Autodesk Inventor part; units mm, degrees
ref_plane "YZ Plane" through (0, 0, 0) normal (1, 0, 0) x (0, 1, 0)
ref_plane "XZ Plane" through (0, 0, 0) normal (0, 1, 0) x (-1, 0, 0)
ref_plane "XY Plane" through (0, 0, 0) normal (0, 0, 1) x (1, 0, 0)
sketch "Skizze1" plane through (0, 0, 0) normal (0, 1, 0) x (-1, 0, 0)
  line L0 (0, 0) -> (32, 0)
  line L1 (32, 0) -> (32, 5)
  line L2 (32, 5) -> (0, 5)
  line L3 (0, 5) -> (0, 0)
  dimension "d0" = 32
  dimension "d1" = 5
extrude "Extrusion1" add sketch "Skizze1" along normal blind 2
ref_plane "Arbeitsebene1" through (-32, 0, 2.5) normal (0, 0, 1) x (1, 0, 0)
ref_plane "Arbeitsebene2" through (-16, 0, 5) normal (1, 0, 0) x (0, 0, -1)
sketch "Skizze2" plane through (0, 2, 0) normal (0, 1, 0) x (1, 0, 0)
  line L0 (6.4, -2.5) -> (-38.4, -2.5)
  line L1 (-16, 1) -> (-16, -6)
  point P0 (0, 0)
  point P1 (-28.5, -2.5)
  point P2 (-16, -2.5)
  point P3 (-3.5, -2.5)
  dimension "d4" = 25
  dimension "d5" = 12.5
hole "Bohrung1" at (-28.5, 2, 2.5) at (-16, 2, 2.5) at (-3.5, 2, 2.5) direction (0, -1, 0) diameter 3.2 end through all
sketch "Skizze3" plane through (0, 2, 0) normal (0, 1, 0) x (1, 0, 0)
  line L0 (-18, -4.75) -> (-25, -4.75)
  line L1 (-25, -4.75) -> (-25, -4.25)
  line L2 (-25, -4.25) -> (-18, -4.25)
  line L3 (-18, -4.25) -> (-18, -4.75)
  line L4 (-18, -3.75) -> (-25, -3.75)
  line L5 (-25, -3.75) -> (-25, -3.25)
  line L6 (-25, -3.25) -> (-18, -3.25)
  line L7 (-18, -3.25) -> (-18, -3.75)
  line L8 (-18, -2.75) -> (-25, -2.75)
  line L9 (-25, -2.75) -> (-25, -2.25)
  line L10 (-25, -2.25) -> (-18, -2.25)
  line L11 (-18, -2.25) -> (-18, -2.75)
  line L12 (-18, -1.75) -> (-25, -1.75)
  line L13 (-25, -1.75) -> (-25, -1.25)
  line L14 (-25, -1.25) -> (-18, -1.25)
  line L15 (-18, -1.25) -> (-18, -1.75)
  line L16 (-18, -0.75) -> (-25, -0.75)
  line L17 (-25, -0.75) -> (-25, -0.25)
  line L18 (-25, -0.25) -> (-18, -0.25)
  line L19 (-18, -0.25) -> (-18, -0.75)
  line L20 (-16, 1) -> (-16, -6)
  line L21 (-32, -5) -> (0, -5)
  line L22 (0, 0) -> (-32, 0)
  dimension "d13" = 2
  dimension "d14" = 7
  dimension "d15" = 0.5
  dimension "d16" = 0.5
  dimension "d17" = 0.5
  dimension "d18" = 0.5
  dimension "d19" = 0.5
  dimension "d20" = 0.25
  dimension "d21" = 0.25
extrude "Extrusion2" add sketch "Skizze3" along normal blind 0.2
fillet "Rundung1" radius 0.25 10 edges at (-21.5, 2.2, 4.25) (-21.5, 2.2, 4.75) (-21.5, 2.2, 3.75) (-21.5, 2.2, 3.25) (-21.5, 2.2, 2.75) (-21.5, 2.2, 2.25) (-21.5, 2.2, 1.75) (-21.5, 2.2, 1.25) (-21.5, 2.2, 0.75) (-21.5, 2.2, 0.25)
mirror "Spiegeln1" about plane through (-16, 0, 5) normal (1, 0, 0) of "Rundung1", "Extrusion2"
chamfer "Fase1" distance 0.25 angle 45 4 edges at (-16, 2, 5) (-16, 2, 0) (0, 2, 2.5) (-32, 2, 2.5)
fillet "Rundung2" radius 1 4 edges at (-32, 0.875, 5) (-32, 0.875, 0) (0, 0.875, 5) (0, 0.875, 0)
equation "\"d16\" = d15"
equation "\"d17\" = d16"
equation "\"d18\" = d17"
equation "\"d19\" = d17"
properties part number "x_carriage_aio_clamp"
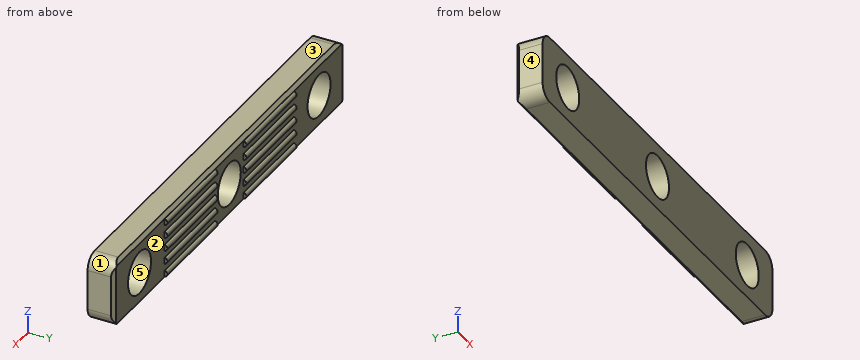
Can you work these out from the model? Positions are in its coordinate system, mm. Face numbers are marked on the shaded views. A direction names the side the tool comes from. Give positions to 0.01 mm unless a question says otherwise; leave off trailing zeros. Loops run counter-clockwise (first coordinate to the right, second up) from the corner with the lowest first, then second, coordinate; pieces in that order, holes last. Notation, with made-up numbers: M -8.5,89 L 1.5,89 A23 ccw 1.5,106 Z; hole C 58,-6 d3. An arc over 180 degrees is marked long. Answer in a Markdown table with one row per item.
1. Suppose I cut it at B-B on y = 0.95. Write out the boundary of the cut face in (x, z), plus the area to 3 significant figures.
Taken from the geometry:
| item | result |
|---|---|
| outline | M -32,1 A1 ccw -31,0 L -1,0 A1 ccw 0,1 L 0,4 A1 ccw -1,5 L -31,5 A1 ccw -32,4 Z; hole C -28.5,2.5 d3.2; hole C -16,2.5 d3.2; hole C -3.5,2.5 d3.2 |
| area | 135 mm² |
2. For pin 1 Ø1.9 at (x, z) = (-28.5, 2.5) entering from +Y; pin 2 Ø1 at (x, z) = (-11.5, 1) entering from +Y; pin 3 Ø1 at (x, z) = (-3.5, 4) entering from +Y, each with a flat end and sliding along its axis, tell me the tip position at first contact or that it passes through.
Taken from the geometry:
| item | result |
|---|---|
| pin 1 | passes through |
| pin 2 | stops at y = 2.2 |
| pin 3 | stops at y = 2 |
3. Thinking about a two-plate mould opening in Z: for the marked faces 3, 4 and 5, which applies, released by +Z, released by -Z, zero draft, split by the parting line, or undercut?
Taken from the geometry:
| item | result |
|---|---|
| face 3 | released by +Z |
| face 4 | zero draft |
| face 5 | undercut |
4. Suppose I cut it at A-A on x = -28.5. Write out the boundary of the cut face in (y, z).
Taken from the geometry:
| item | result |
|---|---|
| outline | M 0,0 L 1.75,0 L 2,0.25 L 2,0.9 L 0,0.9 Z; M 0,4.1 L 2,4.1 L 2,4.75 L 1.75,5 L 0,5 Z |
5. Which directions (+Z, -Z, +X, -X, +Y, -Y) give clear straight access to the entire face, cutting with the end or side of a thin tool? Please do the marked faces 1 and 2.
Taken from the geometry:
| item | result |
|---|---|
| face 1 | +Z, +X, +Y, -Y |
| face 2 | +Y |
6. If I drill on line 1 along X through (y, z) = (0.95, 2.5); line 2 along Z through (x, y) = (-3.5, 1.1); line 3 along X through (y, z) = (0.3, 3.35), over which ranges is the centre line in solid material (lowest first)?
Taken from the geometry:
| item | result |
|---|---|
| line 1 | x = -32 to -30.1, -26.9 to -17.6, -14.4 to -5.1, -1.9 to 0 |
| line 2 | z = 0 to 0.9, 4.1 to 5 |
| line 3 | x = -32 to -29.86, -27.14 to -17.36, -14.64 to -4.86, -2.14 to 0 |
